Geometry: see drawing. Coordinates: mm, zero at the bounding-box minimum. Coordinates: 2 decimals unless noted, no trailing zeros. Write each loop counter-clockwise with the first axis right and the second up, starting at its lowest first coordinate (ties: lowest second). Pieces come first, ordered by that corner, then holes. Notation, with made-up numbers: (-36.75, 24.5) -> (4.25, 24.5) arc R11 ccw to (4.25, 36.5) -> close; hole circle Ø5 at (-21.5, -0.5). An arc over 180 degrees is marked (long way). Use one line per item in the form item = value. Start each with the question number.
(1) Cut plane B-B on z = 14.5. Return the cut outline in (x, y).
(2) Ray query, line 1 along Z through (x, y) = (9, 3.75); line 2 along Z through (x, y) = (2.25, 7.75); line 3 along Z through (x, y) = (10, 2.5). Return the intervals inside material, ascending.
(3) Pull-direction query (Z, two-part tool) for the marked faces 1, 2, 3 and 4; classes: released by +Z, released by -Z, zero draft, split by the parting line, or undercut.
(4) Cut plane A-A on x = 9. Return the cut outline in (y, z), plus the area to 3 significant figures.
(5) First-contact query: pin 1 (2 mm diameter, centred on x = 4, y = 3, fed in from -Z); pin 2 (10 mm diameter, centred on x = 11, z = 14, fed in from +Y); pin 3 (1.3 mm diameter, centred on x = 8, z = 1, fed in from -Y). Flat tips, straight axial feed; report the tip coordinate or a pass-through.
(6) Cut plane D-D on x = 14.5. Return the cut outline in (y, z).
(7) Cut plane C-C on y = 5.25. Return the cut outline in (x, z), plus the area to 3 significant figures.
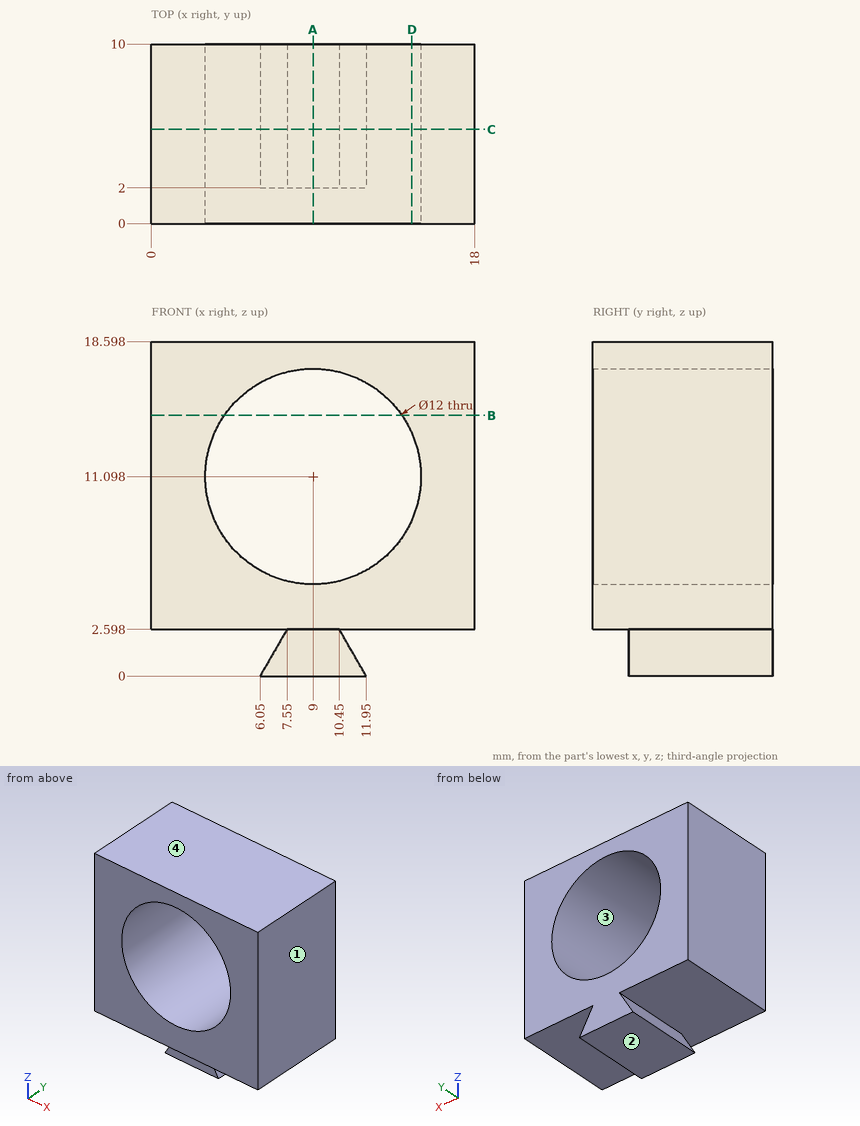
Values:
q1.outline = (0, 0) -> (4.06, 0) -> (4.06, 10) -> (0, 10) -> close; (13.94, 0) -> (18, 0) -> (18, 10) -> (13.94, 10) -> close
q2.line_1 = 0 to 5.1, 17.1 to 18.6
q2.line_2 = 2.6 to 18.6
q2.line_3 = 0 to 5.18, 17.01 to 18.6
q3.face_1 = zero draft
q3.face_2 = released by -Z
q3.face_3 = undercut
q3.face_4 = released by +Z
q4.outline = (0, 2.6) -> (2, 2.6) -> (2, 0) -> (10, 0) -> (10, 5.1) -> (0, 5.1) -> close; (0, 17.1) -> (10, 17.1) -> (10, 18.6) -> (0, 18.6) -> close
q4.area = 60.8 mm2
q5.pin_1 = 2.6
q5.pin_2 = 10
q5.pin_3 = 2
q6.outline = (0, 2.6) -> (10, 2.6) -> (10, 8.7) -> (0, 8.7) -> close; (0, 13.5) -> (10, 13.5) -> (10, 18.6) -> (0, 18.6) -> close
q7.outline = (0, 2.6) -> (7.55, 2.6) -> (6.05, 0) -> (11.95, 0) -> (10.45, 2.6) -> (18, 2.6) -> (18, 18.6) -> (0, 18.6) -> close; hole circle Ø12 at (9, 11.1)
q7.area = 186 mm2
